Could you check a few things on this model? Use its own coordinates, in mm. Face numbers are marked on the shaded views. A direction names the side the tool comes from. Coordinates: 2 decimals unless noted, no trailing zeros. Write each loop counter-clockwise with the first axis right and the second up, starting at its lowest first coordinate (ties: lowest second). Pieces come first, ordered by that corner, then holes.
Item 1: I want a section at A-A on y = 0. Please give me the cut outline in (x, z), then the cut area to 3 significant figures.
Item 2: If I drill on probe 1 along Y at (x, z) = (0, 0.9); probe 2 along Y at (x, z) = (2.5, -2.4); probe 3 along X at (y, z) = (2.5, -2.1), over which ranges is the centre line in solid material (lowest first)?
Item 3: I want a section at B-B on z = -2.4. Please give me the cut outline in (x, y) (3 decimals).
Item 4: For P1, Ø1, axis at y = 4, z = -0.5, coming from the +X side; P2, Ø0.7, axis at y = 2.5, z = -2.5, coming from the +X side; P3, Ø1.5, axis at y = -1.5, z = 1, coming from the -X side, each with a flat end and sliding along its axis, tell me the tip position at first contact or that it passes through.
Item 5: Which directions (+Z, -Z, +X, -X, +Y, -Y) give clear straight access to the entire face, cutting with the end or side of a thin tool? Please do the marked faces 4 and 5.
Item 6: I want a section at D-D on y = 4.25. Please give me the cut outline in (x, z), then the cut area to 3 significant figures.
Item 7: I want a section at C-C on x = 1.75. Please give me the cut outline in (y, z), then the cut area to 3 significant figures.
Item 8: Thinking about a two-plate mould opening in Y: for the marked faces 1, 2 and 3, which applies, +Y half, -Y half, draft (parallel to the pull), parting line (faces both ways), or undercut?
from build123d import *

# Parameters (mm, degrees)
SKETCH1_R           = 7.05
SKETCH1_R_2         = 5.05
SKETCH1_R_3         = 3.05
BOSS_EXTRUDE1_DEPTH = 2
BOSS_EXTRUDE2_START = -3.5
SKETCH1_3_R         = 7.05
SKETCH1_3_R_2       = 5.05
BOSS_EXTRUDE2_DEPTH = 3.5
CUT_EXTRUDE1_DEPTH  = 3.5


with BuildPart() as part:
    # Sketch1 → Boss-Extrude1 (new body)
    # profile 1 of 2: a face of its own
    with BuildSketch(Plane.XY):
        Circle(SKETCH1_R)
        Circle(SKETCH1_R_2, mode=Mode.SUBTRACT)
    # profile 2 of 2: a face of its own
    with BuildSketch(Plane.XY):
        Circle(SKETCH1_R_2)
        Circle(SKETCH1_R_3, mode=Mode.SUBTRACT)
    extrude(amount=BOSS_EXTRUDE1_DEPTH)

    # Sketch1<3> → Boss-Extrude2 (add)
    with BuildSketch(Plane.XY.offset(BOSS_EXTRUDE2_START)):
        Circle(SKETCH1_3_R)
        Circle(SKETCH1_3_R_2, mode=Mode.SUBTRACT)
    extrude(amount=BOSS_EXTRUDE2_DEPTH)

    # Sketch2 → Cut-Extrude1 (cut)
    with BuildSketch(Plane(origin=(0, 0, -3.5), x_dir=(-1, 0, 0), z_dir=(0, 0, -1))):
        with BuildLine():
            Line((0.576871206, 5.016943254), (0, 5.35))
            Line((0, 5.35), (-0.576871206, 5.016943254))
            ThreePointArc((-0.576871206, 5.016943254), (0, 5.05), (0.576871206, 5.016943254))
        make_face()
        with BuildLine():
            Line((4.63323591, 2.675), (4.056364704, 3.008056746))
            ThreePointArc((4.056364704, 3.008056746), (4.373428289, 2.525), (4.63323591, 2.008886507))
            Line((4.63323591, 2.008886507), (4.63323591, 2.675))
        make_face()
        with BuildLine():
            ThreePointArc((-4.63323591, 2.008886507), (-4.373428289, 2.525), (-4.056364704, 3.008056746))
            Line((-4.056364704, 3.008056746), (-4.63323591, 2.675))
            Line((-4.63323591, 2.675), (-4.63323591, 2.008886507))
        make_face()
        with BuildLine():
            ThreePointArc((-4.056364704, -3.008056746), (-4.373428289, -2.525), (-4.63323591, -2.008886507))
            Line((-4.63323591, -2.008886507), (-4.63323591, -2.675))
            Line((-4.63323591, -2.675), (-4.056364704, -3.008056746))
        make_face()
        with BuildLine():
            ThreePointArc((0.576871206, -5.016943254), (0, -5.05), (-0.576871206, -5.016943254))
            Line((-0.576871206, -5.016943254), (0, -5.35))
            Line((0, -5.35), (0.576871206, -5.016943254))
        make_face()
        with BuildLine():
            Line((4.63323591, -2.675), (4.63323591, -2.008886507))
            ThreePointArc((4.63323591, -2.008886507), (4.373428289, -2.525), (4.056364704, -3.008056746))
            Line((4.056364704, -3.008056746), (4.63323591, -2.675))
        make_face()
    extrude(amount=-CUT_EXTRUDE1_DEPTH, mode=Mode.SUBTRACT)


solid = part.part
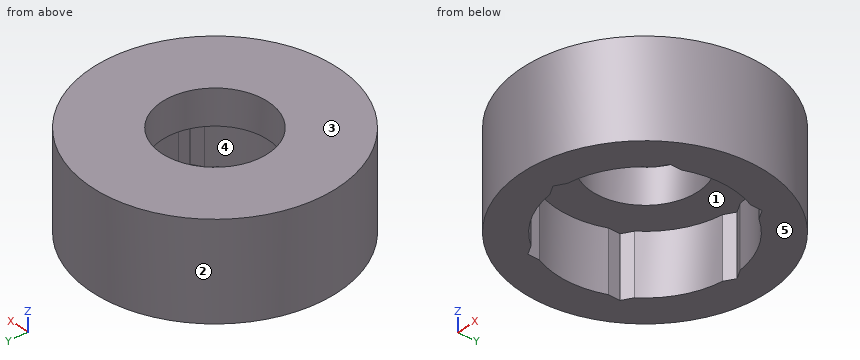
Response values:
1. outline: (-7.05, -3.5) - (-5.05, -3.5) - (-5.05, 0) - (-3.05, 0) - (-3.05, 2) - (-7.05, 2) - close; (3.05, 0) - (5.05, 0) - (5.05, -3.5) - (7.05, -3.5) - (7.05, 2) - (3.05, 2) - close
1. area: 30.0 mm2
2. probe 1: y = -7.05 to -3.05, 3.05 to 7.05
2. probe 2: y = -6.59 to -4.39, 4.39 to 6.59
2. probe 3: x = -6.59 to -4.63, 4.63 to 6.59
3. outline: circle Ø14.1 at (0, 0); hole (-4.633, -2.675) - (-4.056, -3.008) arc R5.05 ccw to (-0.577, -5.017) - (0, -5.35) - (0.577, -5.017) arc R5.05 ccw to (4.056, -3.008) - (4.633, -2.675) - (4.633, -2.009) arc R5.05 ccw to (4.633, 2.009) - (4.633, 2.675) - (4.056, 3.008) arc R5.05 ccw to (0.577, 5.017) - (0, 5.35) - (-0.577, 5.017) arc R5.05 ccw to (-4.056, 3.008) - (-4.633, 2.675) - (-4.633, 2.009) arc R5.05 ccw to (-4.633, -2.009) - close
4. P1: stops at x = 6.12
4. P2: stops at x = 6.71
4. P3: stops at x = -7.01
5. face 4: -Z
5. face 5: -Z, +X, -X, +Y, -Y
6. outline: (-5.62, -3.5) - (-2.73, -3.5) - (-2.73, 0) - (2.73, 0) - (2.73, -3.5) - (5.62, -3.5) - (5.62, 2) - (-5.62, 2) - close
6. area: 42.8 mm2
7. outline: (-6.83, -3.5) - (-4.74, -3.5) - (-4.74, 0) - (-2.5, 0) - (-2.5, 2) - (-6.83, 2) - close; (2.5, 0) - (4.74, 0) - (4.74, -3.5) - (6.83, -3.5) - (6.83, 2) - (2.5, 2) - close
7. area: 32.0 mm2
8. face 1: undercut
8. face 2: parting line
8. face 3: draft
